Source: three-view drawing plus pictorial views. Frame: mm from the lowest corner of the part. A direction names the side the tool comes from. Give positions to 0.01 mm unless a question says otherwise; leave off trailing zeros. Write each loop counter-clockwise with the first axis right and the second up, starting at its lowest first coordinate (ties: lowest second). Pieces come first, ordered by that corner, then holes.
Q1. Line query: L1, parallel to Z at x = 12, y = 35; L2, parallel to X at y = 20.5, z = 27. Output: solid intervals per line, ascending.
Q2. Cut plane C-C on z = 2.5. Return the cut outline in (x, y).
Q3. Cut plane B-B on x = 15.5. Return the cut outline in (y, z).
Q4. Reachability of the marked faces 4, 5, 6, 7 and 8 from +Z, -Z, +X, -X, +Y, -Y: full face, straight path, thin tool, end or side. Return the list, or none.
Q5. Pin query (flat end, axial travel): pin 1 (2.5 mm diameter, centred on y = 25, z = 28, fed in from +X); pin 2 (2.5 mm diameter, centred on x = 28, y = 37, fed in from +Z); pin 3 (2 mm diameter, centred on y = 41, z = 10.5, fed in from +X). Return the tip coordinate at first contact, or that it passes through.
Q6. Draft query along X for the marked faces 1, 2 and 3. Return one class per face: pulls with the +X half, pulls with the -X half, needs draft (parallel to the pull), parting line crosses it, or undercut.
Q7. Cut plane A-A on z = 15.5. Return the cut outline in (x, y), plus the area to 3 significant figures.
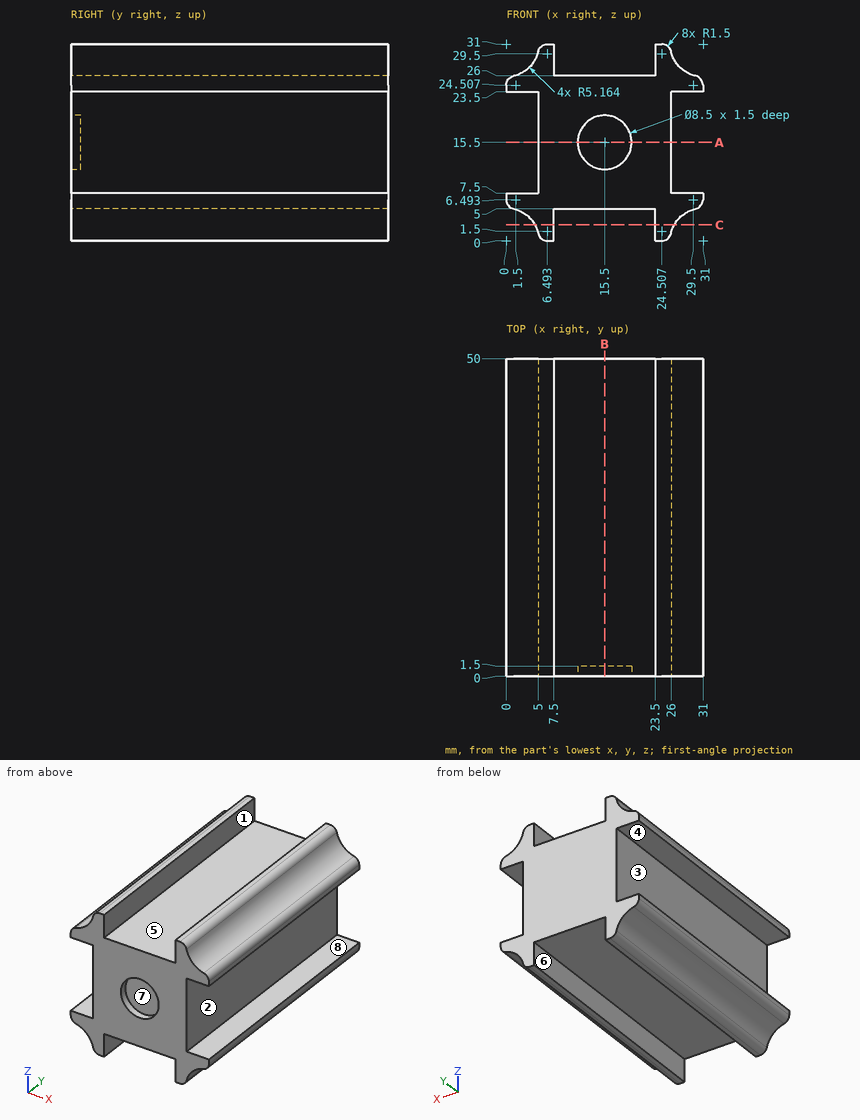
Data:
1. L1: z = 5 to 26
1. L2: x = 3.27 to 7.5, 23.5 to 27.73
2. outline: (4.52, 0) - (7.5, 0) - (7.5, 50) - (4.52, 50) - close; (23.5, 0) - (26.48, 0) - (26.48, 50) - (23.5, 50) - close
3. outline: (0, 5) - (50, 5) - (50, 26) - (0, 26) - (0, 19.75) - (1.5, 19.75) - (1.5, 11.25) - (0, 11.25) - close
4. face 4: -X, +Y, -Y
4. face 5: +Z, +Y, -Y
4. face 6: -Z, +Y, -Y
4. face 7: -Y
4. face 8: +X, +Y, -Y
5. pin 1: stops at x = 28.07
5. pin 2: stops at z = 28.07
5. pin 3: stops at x = 26
6. face 1: undercut
6. face 2: pulls with the +X half
6. face 3: pulls with the -X half
7. outline: (5, 0) - (11.25, 0) - (11.25, 1.5) - (19.75, 1.5) - (19.75, 0) - (26, 0) - (26, 50) - (5, 50) - close
7. area: 1,040 mm2
